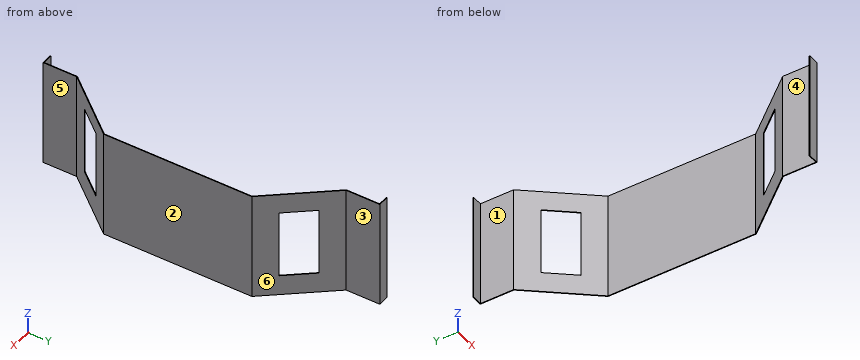
```python
from build123d import *

# Parameters (mm, degrees)
BOSS_EXTRUDE1_DEPTH = 159
SKETCH2_W           = 100
SKETCH2_H           = 50
CUT_EXTRUDE1_DEPTH  = 160
SKETCH5_W           = 100
SKETCH5_H           = 50
CUT_EXTRUDE2_DEPTH  = 160


with BuildPart() as part:
    # Sketch1 → Boss-Extrude1 (new body)
    with BuildSketch(Plane.XY):
        Polygon((0, 110), (0, -110), (-75, -200), (-75, -249), (-75, -250), (-91, -250), (-91, -249), (-76, -249), (-76, -199.637950065), (-1, -109.637950065), (-1, 109.637950065), (-76, 199.637950065), (-76, 249), (-91, 249), (-91, 250), (-75, 250), (-75, 249), (-75, 200), align=None)
    extrude(amount=BOSS_EXTRUDE1_DEPTH)

    # Sketch2 → Cut-Extrude1 (cut)
    with BuildSketch(Plane(origin=(54.098360656, -45.081967213, 0), x_dir=(0, 0, -1), z_dir=(0.76822128, -0.6401844, 0))):
        with Locations((-84, -143.004340756)):
            Rectangle(SKETCH2_W, SKETCH2_H)
    extrude(amount=-CUT_EXTRUDE1_DEPTH, mode=Mode.SUBTRACT)

    # Sketch5 → Cut-Extrude2 (cut)
    with BuildSketch(Plane(origin=(54.098360656, 45.081967213, 0), x_dir=(0, 0, -1), z_dir=(0.76822128, 0.6401844, 0))):
        with Locations((-80, 143.158085894)):
            Rectangle(SKETCH5_W, SKETCH5_H)
    extrude(amount=-CUT_EXTRUDE2_DEPTH, mode=Mode.SUBTRACT)


solid = part.part
```
Geometry: final body of the model. Coordinates: model frame, mm. Face numbers are marked on the shaded views. A direction names the side the tool comes from. Round coordinates to 2 decimals unless told otherwise and drop trailing zeros. Order: outer loops, then holes, each group sorted by start corner. A loop starts at its lowest first (then second) coordinate and runs counter-clockwise, first axis right, second up. Notation, with made-up numbers: (65, 38) -> (95, 38) arc R20 ccw to (95, 73) -> close; hole circle Ø8 at (9.25, 42.25). An arc over 180 degrees is marked (long way). Write each question's results on one line, items separated by ' | '.
Q1. Section query A-A (z = 112). Output: boundary loops of the cut face in (x, y), and give its area (3 significant figures).
Response values:
outline: (-91, -250) -> (-75, -250) -> (-75, -200) -> (-53.46, -174.15) -> (-54.22, -173.51) -> (-76, -199.64) -> (-76, -249) -> (-91, -249) -> close; (-91, 249) -> (-76, 249) -> (-76, 199.64) -> (-54.32, 173.62) -> (-53.55, 174.26) -> (-75, 200) -> (-75, 250) -> (-91, 250) -> close; (-22.31, 135.21) -> (-1, 109.64) -> (-1, -109.64) -> (-22.21, -135.1) -> (-21.45, -135.74) -> (0, -110) -> (0, 110) -> (-21.54, 135.85) -> close | area: 484 mm²
Q2. Section query B-B (x = -42). Output: boundary loops of the cut face in (y, z).
Response values:
outline: (-160.4, 0) -> (-158.84, 0) -> (-158.84, 34) -> (-160.4, 34) -> close; (-160.4, 134) -> (-158.84, 134) -> (-158.84, 159) -> (-160.4, 159) -> close; (158.84, 0) -> (160.4, 0) -> (160.4, 30) -> (158.84, 30) -> close; (158.84, 130) -> (160.4, 130) -> (160.4, 159) -> (158.84, 159) -> close
Q3. Section query C-C (z = 139.5). Output: boundary loops of the cut face in (x, y), and give its area (3 significant figures).
Response values:
outline: (-91, -250) -> (-75, -250) -> (-75, -200) -> (0, -110) -> (0, 110) -> (-75, 200) -> (-75, 250) -> (-91, 250) -> (-91, 249) -> (-76, 249) -> (-76, 199.64) -> (-1, 109.64) -> (-1, -109.64) -> (-76, -199.64) -> (-76, -249) -> (-91, -249) -> close | area: 584 mm²
Q4. Access query for the marked faces 1, 2 and 3. Directions: +Z, -Z, +X, -X, +Y, -Y. A direction counts if a zero-diameter tool reaches every point of the face in a straight line with its end or side. Return the directions, or none.
Response values:
face 1: +Z, -Z, -X | face 2: +Z, -Z, +X, +Y, -Y | face 3: +Z, -Z, +X, +Y
Q5. Pin query (flat end, axial travel): pin 1 Ø4 at (x, z) = (-70.5, 109) entering from +Y; pin 2 Ø4 at (y, z) = (166.5, 16.5) entering from +X; pin 3 Ø24.5 at (y, z) = (220.5, 103) entering from -X. Return the tip coordinate at first contact, or that it passes through.
Response values:
pin 1: y = 197 | pin 2: x = -45.42 | pin 3: x = -76
Q6. Ray query, line 1 along X through (y, z) = (7.5, 8); line 2 along Y through (x, z) = (-79, 125.5); line 3 along X through (y, z) = (-221.5, 117.5). Return the intervals inside material, ascending.
Response values:
line 1: -1 to 0 | line 2: -250 to -249, 249 to 250 | line 3: -76 to -75
Q7. Section query D-D (x = -16.5). Output: boundary loops of the cut face in (y, z).
Response values:
outline: (-129.8, 0) -> (-128.24, 0) -> (-128.24, 159) -> (-129.8, 159) -> close; (128.24, 0) -> (129.8, 0) -> (129.8, 159) -> (128.24, 159) -> close
Q8. Pull-direction query (Y, two-part tool) for the marked faces 4, 5 and 6; classes: released by +Y, released by -Y, zero draft, split by the parting line, or undercut.
Response values:
face 4: undercut | face 5: zero draft | face 6: released by +Y
